from build123d import *

# Parameters (mm, degrees)
SKETCH1_R           = 6.25
BOSS_EXTRUDE1_DEPTH = 15
SKETCH3_R           = 7.5
BOSS_EXTRUDE2_DEPTH = 35
SKETCH4_R           = 5
CUT_EXTRUDE1_DEPTH  = 25
SKETCH5_R           = 2.5
CUT_EXTRUDE2_DEPTH  = 35


with BuildPart() as part:
    # Sketch1 → Boss-Extrude1 (new body)
    with BuildSketch(Plane(origin=(0, 0, 0), x_dir=(1, 0, 0), z_dir=(0, 1, 0))):
        Circle(SKETCH1_R)
    extrude(amount=BOSS_EXTRUDE1_DEPTH)

    # Sketch3 → Boss-Extrude2 (add)
    with BuildSketch(Plane(origin=(0, 15, 0), x_dir=(1, 0, 0), z_dir=(0, 1, 0))):
        Circle(SKETCH3_R)
    extrude(amount=BOSS_EXTRUDE2_DEPTH)

    # Sketch4 → Cut-Extrude1 (cut)
    with BuildSketch(Plane(origin=(0, 50, 0), x_dir=(1, 0, 0), z_dir=(0, 1, 0))):
        Circle(SKETCH4_R)
    extrude(amount=-CUT_EXTRUDE1_DEPTH, mode=Mode.SUBTRACT)

    # Sketch5 → Cut-Extrude2 (cut)
    with BuildSketch(Plane(origin=(0, 0, 0), x_dir=(-1, 0, 0), z_dir=(0, -1, 0))):
        Circle(SKETCH5_R)
    extrude(amount=-CUT_EXTRUDE2_DEPTH, mode=Mode.SUBTRACT)


solid = part.part
Design review of the part built by this model. Coordinates are the model's own, in mm. A direction names the side the tool comes from. Coordinates: 2 decimals unless noted, no trailing zeros. Order: outer loops, then holes, each group sorted by start corner. A loop starts at its lowest first (then second) coordinate and runs counter-clockwise, first axis right, second up.
Item 1: Take a section at D-D, the plane x = 3.25. Write out the cut boundary in (y, z), then the cut area to 3 significant figures.
Item 2: Take a section at A-A, the plane x = 0. Write out the cut boundary in (y, z), then the cut area to 4 significant figures.
Item 3: Take a section at C-C, the plane y = 30. Write out the cut boundary in (x, z), then the cut area to 3 significant figures.
Item 4: For faces 4 (the cylindrical face through (-1.08, 37.67, 4.88)), 5 (the cylindrical face through (5.96, 7.4, -1.88)), 6 (the flat face through (0, 0, 3)), list the 3-axis set-ups (+Z, -Z, +X, -X, +Y, -Y) from which the entire face can be reached by the end or side of a thin tool; tool diameter is ignored.
Item 5: Take a section at B-B, the plane z = 0. Write out the cut boundary in (x, y).
Item 6: For pin 1 Ø2 at (x, y) = (1.5, 23) entering from +Z; pin 2 Ø8 at (x, z) = (0, 0) entering from +Y; pin 3 Ø4 at (x, y) = (-4, 8.5) entering from -Z, all flat-tipped, find the tip position at first contact; note any pin that passes through.
Item 7: For line 1 (Z direction, x = 0, y = 10.25); line 2 (Z direction, x = 0, y = 45.25), list the stretches that pass through material, from the lowest coordinate up.
Item 8: The part is to be moulded in two halves that separate along Z. For faces 1 (the cylindrical face through (0.54, 12.32, 2.44)), 2 (the flat face through (-3, 15, -6)), 3 (the cylindrical face through (-7.493, 32.255, -0.33)), say which applies: pulls with the +Z half, pulls with the -Z half, needs draft (parallel to the pull), parting line crosses it, or undercut.
The answers:
1. outline: (0, -5.34) - (15, -5.34) - (15, -6.76) - (50, -6.76) - (50, -3.8) - (25, -3.8) - (25, 3.8) - (50, 3.8) - (50, 6.76) - (15, 6.76) - (15, 5.34) - (0, 5.34) - close
1. area: 443 mm2
2. outline: (0, -6.25) - (15, -6.25) - (15, -7.5) - (50, -7.5) - (50, -5) - (25, -5) - (25, -2.5) - (0, -2.5) - close; (0, 2.5) - (25, 2.5) - (25, 5) - (50, 5) - (50, 7.5) - (15, 7.5) - (15, 6.25) - (0, 6.25) - close
2. area: 337.5 mm2
3. outline: circle Ø15 at (0, 0); hole circle Ø10 at (0, 0)
3. area: 98.2 mm2
4. face 4: +Y
4. face 5: -Y
4. face 6: +Z, -Z, +X, -X, -Y
5. outline: (-7.5, 15) - (-6.25, 15) - (-6.25, 0) - (-2.5, 0) - (-2.5, 25) - (-5, 25) - (-5, 50) - (-7.5, 50) - close; (2.5, 0) - (6.25, 0) - (6.25, 15) - (7.5, 15) - (7.5, 50) - (5, 50) - (5, 25) - (2.5, 25) - close
6. pin 1: stops at z = 7.48
6. pin 2: stops at y = 25
6. pin 3: stops at z = -5.92
7. line 1: z = -6.25 to -2.5, 2.5 to 6.25
7. line 2: z = -7.5 to -5, 5 to 7.5
8. face 1: undercut
8. face 2: needs draft
8. face 3: parting line crosses it
